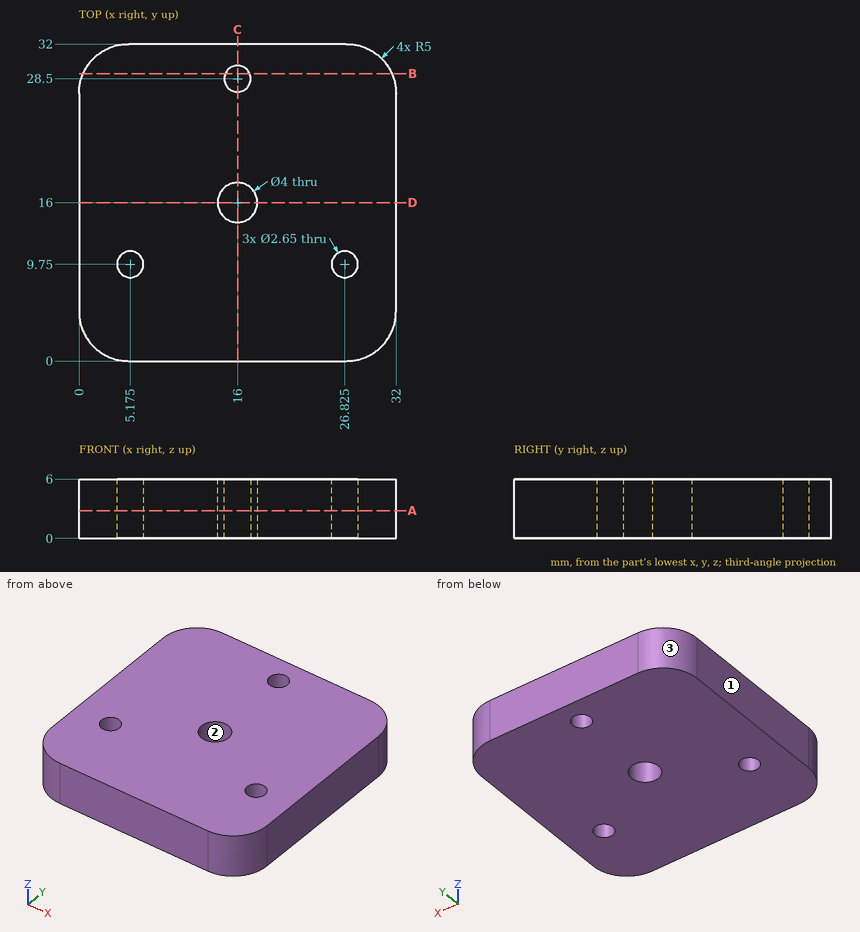
Print and shaded views of the part. All mm, measured from the part's lowest x, y and z. Round coordinates to 2 decimals unless told otherwise and drop trailing zeros. Order: outer loops, then holes, each group sorted by start corner. A loop starts at its lowest first (then second) coordinate and runs counter-clockwise, first axis right, second up.
Q1. Wall check: L1, parallel to Y at x = 16, z = 4 (1 decimal); L2, parallel to X at y = 9, z = 5.7; L3, parallel to Y at x = 17.5, z = 2.9. Give the ranges that are in metal, low to high.
Q2. Drop flat-ended pins along their axis: pin 1 (1.6 mm diameter, centred on x = 26.83, y = 9.75, fed in from -Z); pin 2 (1.5 mm diameter, centred on y = 29, z = 1, fed in from +X); pin 3 (1.5 mm diameter, centred on x = 3.5, z = 0.5, fed in from -Y). Give the stop position or say it passes through.
Q3. Two-plate mould, pull along Y, no slides. Class the marked faces 1, 2 and 3: pulls with the +Y half, pulls with the -Y half, needs draft (parallel to the pull), parting line crosses it, or undercut.
Q4. Slice it at D-D (y = 16). Write the cut outline in (x, z), and give its area (3 significant figures).
Q5. Slice it at C-C (x = 16). Write the cut outline in (y, z) (1 decimal).
Q6. Slice it at B-B (y = 29). Write the cut outline in (x, z).
Q7. Slice it at A-A (z = 2.8). State how many separate pieces and enclosed holes the cut face has.
Results below:
1. L1: y = 0 to 14, 18 to 27.2, 29.8 to 32
1. L2: x = 0 to 4.08, 6.27 to 25.73, 27.92 to 32
1. L3: y = 0 to 14.68, 17.32 to 32
2. pin 1: passes through
2. pin 2: stops at x = 31.84
2. pin 3: stops at y = 0.06
3. face 1: needs draft
3. face 2: undercut
3. face 3: pulls with the +Y half
4. outline: (0, 0) - (14, 0) - (14, 6) - (0, 6) - close; (18, 0) - (32, 0) - (32, 6) - (18, 6) - close
4. area: 168 mm2
5. outline: (0, 0) - (14, 0) - (14, 6) - (0, 6) - close; (18, 0) - (27.2, 0) - (27.2, 6) - (18, 6) - close; (29.8, 0) - (32, 0) - (32, 6) - (29.8, 6) - close
6. outline: (0.42, 0) - (14.77, 0) - (14.77, 6) - (0.42, 6) - close; (17.23, 0) - (31.58, 0) - (31.58, 6) - (17.23, 6) - close
7. separate pieces: 1
7. enclosed holes: 4
